from build123d import *

# Parameters (mm, degrees)
BOSS_EXTRUDE1_DEPTH = 8
SKETCH2_W           = 8
SKETCH2_H           = 8
BOSS_EXTRUDE2_DEPTH = 42
SKETCH3_W           = 10
SKETCH3_H           = 5
BOSS_EXTRUDE3_DEPTH = 10
CUT_EXTRUDE1_REACH  = 82.455
SKETCH4_R           = 1.7
CUT_EXTRUDE2_DEPTH  = 2.4
CHAMFER1_SIZE       = 6
MIRROR2_START       = -5
MIRROR2_OUTLINE_W   = 10
MIRROR2_OUTLINE_H   = 10
MIRROR2_DEPTH       = 5
MIRROR2_2_OUTLINE_R = 1.7
MIRROR2_2_DEPTH     = 2.6
MIRROR2_START_2     = -2.4
MIRROR2_3_DEPTH     = 2.4
MIRROR2_4_DEPTH     = 2.4


# Read off the part's stored shape, not the designer's step: Mirror2
with BuildPart() as part:
    # Sketch1 → Boss-Extrude1 (new body)
    with BuildSketch(Plane.XY):
        Polygon((0, 0), (0, 42), (-8, 42), (-8, -8), (42, -8), (42, 0), align=None)
    extrude(amount=BOSS_EXTRUDE1_DEPTH)

    # Sketch2 → Boss-Extrude2 (add)
    with BuildSketch(Plane.XY.offset(8)):
        with Locations((-4, -4)):
            Rectangle(SKETCH2_W, SKETCH2_H)
    extrude(amount=BOSS_EXTRUDE2_DEPTH)

    # Sketch3 → Boss-Extrude3 (add)
    with BuildSketch(Plane.XY.offset(8)):
        with Locations((5, -2.5)):
            Rectangle(SKETCH3_W, SKETCH3_H)
    boss_extrude3 = extrude(amount=BOSS_EXTRUDE3_DEPTH)

    # Sketch4 → Cut-Extrude1 (cut, up to next)
    with BuildSketch(Plane.XZ.offset(5), mode=Mode.PRIVATE) as cut_extrude1_sk1:
        with Locations((5, 13)):
            Circle(SKETCH4_R)
    cut_extrude1_tool1 = extrude(cut_extrude1_sk1.sketch, amount=-CUT_EXTRUDE1_REACH, mode=Mode.PRIVATE) & part.part
    cut_extrude1 = cut_extrude1_tool1.solids().sort_by_distance((5, -5, 13))[0]
    add(cut_extrude1, mode=Mode.SUBTRACT)

    # Sketch5 → Cut-Extrude2 (cut)
    with BuildSketch(Plane(origin=(0, 0, 0), x_dir=(1, 0, 0), z_dir=(0, 1, 0))):
        Polygon((8.464101615, -13), (6.732050808, -10), (3.267949192, -10), (1.535898385, -13), (3.267949192, -16), (6.732050808, -16), align=None)
    cut_extrude2 = extrude(amount=-CUT_EXTRUDE2_DEPTH, mode=Mode.SUBTRACT)

    # Mirror1: Boss-Extrude3, Cut-Extrude1, Cut-Extrude2 across plane
    add(boss_extrude3.mirror(Plane(origin=(0, -4, 4), x_dir=(0, 0.7071067811865489, 0.7071067811865462), z_dir=(0, 0.7071067811865464, -0.7071067811865488))))
    add(cut_extrude1.mirror(Plane(origin=(0, -4, 4), x_dir=(0, 0.7071067811865489, 0.7071067811865462), z_dir=(0, 0.7071067811865464, -0.7071067811865488))), mode=Mode.SUBTRACT)
    add(cut_extrude2.mirror(Plane(origin=(0, -4, 4), x_dir=(0, 0.7071067811865489, 0.7071067811865462), z_dir=(0, 0.7071067811865464, -0.7071067811865488))), mode=Mode.SUBTRACT)

    # Chamfer1
    chamfer1_edges = [part.edges().sort_by_distance(p)[0] for p in [
        (-8, -8, 25),
        (17, -8, 0),
        (-8, 17, 0),
    ]]
    chamfer(chamfer1_edges, length=CHAMFER1_SIZE)

    # Mirror2 outline → Mirror2 (add)
    with BuildSketch(Plane.YZ.offset(MIRROR2_START)):
        with Locations((5, 13)):
            Rectangle(MIRROR2_OUTLINE_W, MIRROR2_OUTLINE_H)
        Polygon((2, 11.267949192), (2, 14.732050808), (5, 16.464101615), (8, 14.732050808), (8, 11.267949192), (5, 9.535898385), align=None, mode=Mode.SUBTRACT)
    extrude(amount=MIRROR2_DEPTH)

    # Mirror2 2 outline → Mirror2 2 (add)
    with BuildSketch(Plane.YZ.offset(MIRROR2_START)):
        Polygon((5, 16.464101615), (2, 14.732050808), (2, 11.267949192), (5, 9.535898385), (8, 11.267949192), (8, 14.732050808), align=None)
        with Locations((5, 13)):
            Circle(MIRROR2_2_OUTLINE_R, mode=Mode.SUBTRACT)
    extrude(amount=MIRROR2_2_DEPTH)

    # Mirror2 3 outline → Mirror2 3 (add)
    with BuildSketch(Plane(origin=(0, 0, 0), x_dir=(1, 0, 0), z_dir=(0, 1, 0)).offset(MIRROR2_START_2)):
        Polygon((6.732050808, -16), (7.196152423, -15.196152423), (5.803847577, -16), align=None)
        Polygon((8, -12.196152423), (8, -13.803847577), (8.464101615, -13), align=None)
        Polygon((3.267949192, -16), (4.196152423, -16), (2.803847577, -15.196152423), align=None)
        Polygon((5.803847577, -10), (7.196152423, -10.803847577), (6.732050808, -10), align=None)
        Polygon((1.535898385, -13), (2, -13.803847577), (2, -12.196152423), align=None)
        Polygon((2.803847577, -10.803847577), (4.196152423, -10), (3.267949192, -10), align=None)
    extrude(amount=MIRROR2_3_DEPTH)

    # Mirror2 4 outline → Mirror2 4 (cut)
    with BuildSketch(Plane(origin=(0, 0, 0), x_dir=(1, 0, 0), z_dir=(0, 1, 0)).offset(MIRROR2_START_2)):
        Polygon((7.196152423, -15.196152423), (8, -14.732050808), (8, -13.803847577), align=None)
        Polygon((5, -16.464101615), (5.803847577, -16), (4.196152423, -16), align=None)
        Polygon((7.196152423, -10.803847577), (8, -12.196152423), (8, -11.267949192), align=None)
        Polygon((2, -14.732050808), (2.803847577, -15.196152423), (2, -13.803847577), align=None)
        Polygon((4.196152423, -10), (5.803847577, -10), (5, -9.535898385), align=None)
        Polygon((2, -11.267949192), (2, -12.196152423), (2.803847577, -10.803847577), align=None)
    extrude(amount=MIRROR2_4_DEPTH, mode=Mode.SUBTRACT)


solid = part.part
The listing builds one solid part. Answer for the finished solid, in the listing's coordinates (mm). A direction names the side the tool comes from. Round coordinates to 2 decimals unless told otherwise and drop trailing zeros. Write each loop counter-clockwise with the first axis right and the second up, starting at its lowest first coordinate (ties: lowest second). Pieces come first, ordered by that corner, then holes. Notation, with made-up numbers: M 10.5,78 L 60.5,78 A32 cw 60.5,114 Z; hole C 0.5,47 d9. An arc over 180 degrees is marked long. Write each question's results on one line, items separated by ' | '. Start each with the question number.
Item 1: Flat-ended cylindrical pins translate along their axes: pin 1 Ø4 at (y, z) = (19.5, 4.5) entering from +X; pin 2 Ø9 at (x, z) = (-3, 18.5) entering from +Y; pin 3 Ø9 at (x, y) = (-3.5, 16) entering from +Z. Find the tip coordinate at first contact, or state that the pin passes through.
Item 2: For faces 1 (the face through (2, -1, 13)), 2 (the face through (4.9, 8.4, 8)), 3 (the face through (7, -5, 13)), 4 (the face through (-1.2, 6.5, 15.6)), determine the directions among +Z, -Z, +X, -X, +Y, -Y from which every point of the face is accessible in a straight line to the end or side of a thin tool.
Item 3: For a pull along Y with two mould halves and no side action, classify faces 5 (the face through (7, 5, 3)), 6 (the face through (-4, -4, 4)), 7 (the face through (-2.4, 4, 15)), 8 (the face through (-1, 8, 13)) as pulls with the +Y half, pulls with the -Y half, needs draft (parallel to the pull), parting line crosses it, or undercut.
Item 4: A cutting plane is placed at A-A on z = 13. Write down the section's boundary in (x, y), and give its area (3 significant figures).
Item 5: Straight lines are drawn through the part: L1, parallel to Y at x = -5, z = 28.5; L2, parallel to Y at x = 35.5, z = 7.5; L3, parallel to Z at x = -4.35, y = 5. For each, find the intervals that lie inside material, in ascending order. Write a range as [from, to].
Item 6: A cutting plane is placed at B-B on x = 26. Write down the section's boundary in (y, z).
Check sheet entries:
1) pin 1: x = 0 | pin 2: y = 10 | pin 3: z = 8
2) face 1: +Y | face 2: +Z, +X, +Y | face 3: +Z, +X, -Y | face 4: +X
3) face 5: needs draft | face 6: pulls with the -Y half | face 7: undercut | face 8: undercut
4) outline: M -8,-2 L -2,-8 L 0,-8 L 0,-5 L 3.3,-5 L 3.3,-2.4 L 2,-2.4 L 2,0 L 0,0 L 0,2 L -2.4,2 L -2.4,3.3 L -5,3.3 L -5,0 L -8,0 Z; M -5,6.7 L -2.4,6.7 L -2.4,8 L 0,8 L 0,10 L -5,10 Z; M 6.7,-5 L 10,-5 L 10,0 L 8,0 L 8,-2.4 L 6.7,-2.4 Z | area: 99.5 mm²
5) L1: [-5, 0] | L2: [-8, 0] | L3: [2.35, 11.3], [14.7, 18]
6) outline: M -8,6 L -2,0 L 0,0 L 0,8 L -8,8 Z
